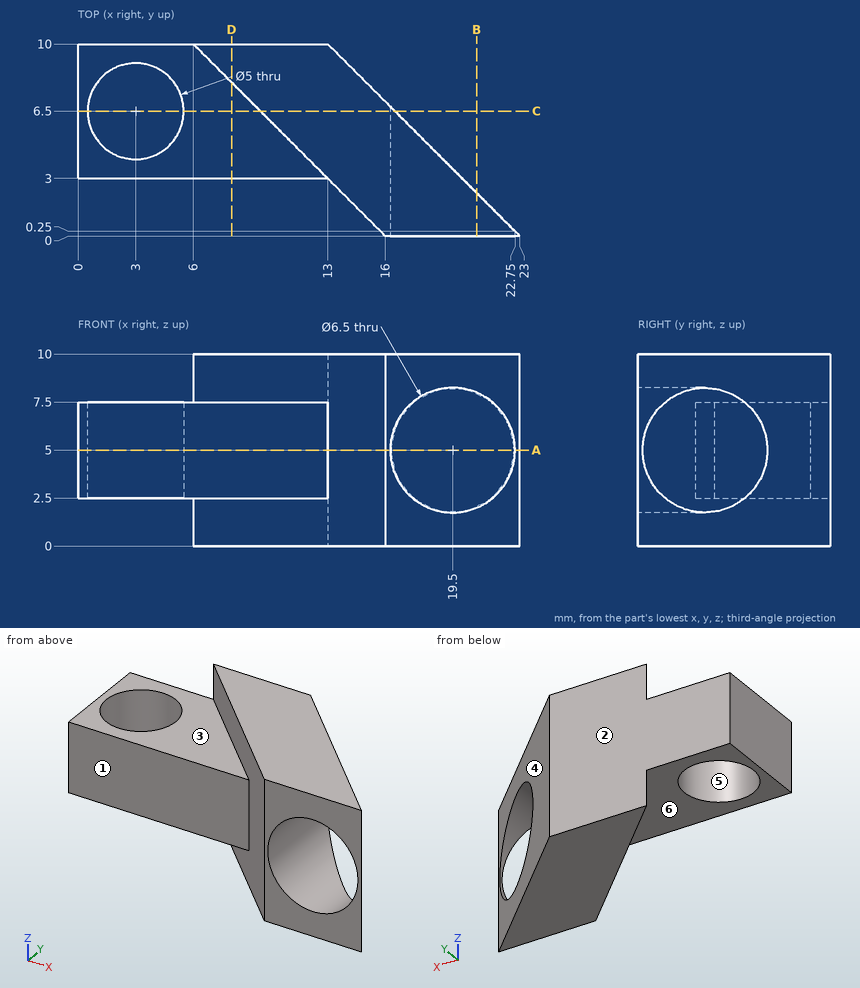
Design review of the part shown in the three views and the two pictorial views. Dimensions are in mm from the part's minimum x, y and z. A direction names the side the tool comes from. Round coordinates to 2 decimals unless told otherwise and drop trailing zeros. Write each loop counter-clockwise with the first axis right and the second up, starting at its lowest first coordinate (ties: lowest second). Pieces come first, ordered by that corner, then holes. Notation, with made-up numbers: (53, 61) - (60, 61) arc R10 ccw to (60, 70) - close; hole circle Ø5 at (29.25, 31). An arc over 180 degrees is marked (long way). Return JSON: item names as keys, results as strings. Group by question number.
Item 1: Machinability: for the marked faces 1, 2 and 3, which of the approach directions +Z, -Z, +X, -X, +Y, -Y give a long, thin tool a straight path to every point of the face, cutting with its end or side? Answer none if there is none.
Item 2: We need section C-C on y = 6.5. Write out the cut boundary in (x, z).
Item 3: The part is to be moulded in two halves that separate along X. For the marked faces 4, 5 and 6, say which applies: pulls with the +X half, pulls with the -X half, needs draft (parallel to the pull), parting line crosses it, or undercut.
Item 4: We need section D-D on x = 8. Write out the cut boundary in (y, z).
Item 5: Insertion check: P1, Ø1, axis at y = 6, z = 6.5, coming from the +X side; P2, Ø1, axis at x = 14.5, z = 5.5, coming from the +Y side; P3, Ø4, axis at x = 4.5, z = 5, coming from the -Y side; P4, Ø2, axis at x = 18.5, y = 6, coming from the -Z side (3 decimals). Each pin has a flat end and moves straight along its axis. Give the tip position at first contact, or say it passes through.
Item 6: We need section B-B on x = 20.75. Write out the cut boundary in (y, z), and give its area (3 significant figures).
Item 7: We need section A-A on z = 5. Write out the cut boundary in (x, y).
Item 8: For probe 1 along Y at (x, z) = (3, 5.2); probe 2 along Z at (x, y) = (19.5, 2.5); probe 3 along Y at (x, z) = (12, 1.75), list the stretches that pass through material, from the lowest coordinate up. Write a range as [from, to].
Model answer:
{
 "1": {"face 1": "+Z, -Z, -X, -Y", "face 2": "+Z, -Z, +X, -X, +Y", "face 3": "+Z, -X, -Y"},
 "2": {"outline": "(0, 2.5) - (0.5, 2.5) - (0.5, 7.5) - (0, 7.5) - close; (5.5, 2.5) - (9.5, 2.5) - (9.5, 0) - (16.5, 0) - (16.5, 3.75) arc R3.25 cw to (16.5, 6.25) - (16.5, 10) - (9.5, 10) - (9.5, 7.5) - (5.5, 7.5) - close"},
 "3": {"face 4": "pulls with the +X half", "face 5": "undercut", "face 6": "needs draft"},
 "4": {"outline": "(3, 2.5) - (8, 2.5) - (8, 0) - (10, 0) - (10, 10) - (8, 10) - (8, 7.5) - (3, 7.5) - close"},
 "5": {"P1": "stops at x = 16.94", "P2": "stops at y = 9", "P3": "stops at y = 3", "P4": "passes through"},
 "6": {"outline": "(0, 0) - (2.25, 0) - (2.25, 2) - (0, 2) - close; (0, 8) - (2.25, 8) - (2.25, 10) - (0, 10) - close", "area": "9.00 mm²"},
 "7": {"outline": "(0, 3) - (13, 3) - (16, 0) - (16.25, 0) - (16.25, 6.75) - (13, 10) - (0, 10) - close; (22.75, 0) - (23, 0) - (22.75, 0.25) - close; hole circle Ø5 at (3, 6.5)"},
 "8": {"probe 1": "y = [3, 4], [9, 10]", "probe 2": "z = [0, 1.75], [8.25, 10]", "probe 3": "y = [4, 10]"}
}
